```python
from build123d import *

# Parameters (mm, degrees)
SKETCH_1_W          = 70
SKETCH_1_H          = 50
SKETCH_1_R          = 1.6
EXTRUDE_1_DEPTH     = 3
SKETCH_2_W          = 30
SKETCH_2_H          = 30
CUT_EXTRUDE_1_DEPTH = 4
FILLET_1_R          = 5
SKETCH_3_W          = 30
SKETCH_3_H          = 6
EXTRUDE_2_DEPTH     = 3
FILLET_2_R          = 3


with BuildPart() as part:
    # 草图1 → 凸台-拉伸1 (new body)
    with BuildSketch(Plane.XY):
        Rectangle(SKETCH_1_W, SKETCH_1_H)
        with Locations((-25, -15)):
            Circle(SKETCH_1_R, mode=Mode.SUBTRACT)
        with Locations((-25, -5)):
            Circle(SKETCH_1_R, mode=Mode.SUBTRACT)
        with Locations((-25, 15)):
            Circle(SKETCH_1_R, mode=Mode.SUBTRACT)
        with Locations((-5, 15)):
            Circle(SKETCH_1_R, mode=Mode.SUBTRACT)
        with Locations((5, 15)):
            Circle(SKETCH_1_R, mode=Mode.SUBTRACT)
        with Locations((25, 15)):
            Circle(SKETCH_1_R, mode=Mode.SUBTRACT)
        with Locations((25, -5)):
            Circle(SKETCH_1_R, mode=Mode.SUBTRACT)
        with Locations((25, -15)):
            Circle(SKETCH_1_R, mode=Mode.SUBTRACT)
    extrude(amount=EXTRUDE_1_DEPTH)

    # 草图2 → 切除-拉伸1 (cut, through all)
    with BuildSketch(Plane.XY.offset(3)):
        with Locations((0, -10)):
            Rectangle(SKETCH_2_W, SKETCH_2_H)
    extrude(amount=-CUT_EXTRUDE_1_DEPTH, mode=Mode.SUBTRACT)

    # 圆角1
    fillet_1_edges = [part.edges().sort_by_distance(p)[0] for p in [
        (15, -25, 1.5),
        (-15, -25, 1.5),
        (-15, 5, 1.5),
        (15, 5, 1.5),
        (35, -25, 1.5),
        (-35, -25, 1.5),
        (-35, 25, 1.5),
        (35, 25, 1.5),
    ]]
    fillet(fillet_1_edges, radius=FILLET_1_R)

    # 草图3 → 凸台-拉伸2 (add)
    with BuildSketch(Plane.XY.offset(3)):
        with Locations((0, -13)):
            Rectangle(SKETCH_3_W, SKETCH_3_H)
    extrude(amount=-EXTRUDE_2_DEPTH)

    # 圆角2
    fillet_2_edges = [part.edges().sort_by_distance(p)[0] for p in [
        (-15, -16, 1.5),
        (-15, -10, 1.5),
        (15, -10, 1.5),
        (15, -16, 1.5),
    ]]
    fillet(fillet_2_edges, radius=FILLET_2_R)


solid = part.part
```
Read the model definition and answer for the solid it produces. Units are mm, in the model's axes. A direction names the side the tool comes from. Coordinates: 2 decimals unless noted, no trailing zeros. Write each loop counter-clockwise with the first axis right and the second up, starting at its lowest first coordinate (ties: lowest second). Pieces come first, ordered by that corner, then holes. Notation, with made-up numbers: (-21.75, 13) -> (20.25, 13) arc R35 cw to (20.25, 50) -> close; hole circle Ø11 at (-9, 24). An arc over 180 degrees is marked (long way). Return JSON: item names as keys, results as strings.
1. Determine the mould class of faces 1 (the face through (25, -25, 1)), 2 (the face through (23.82, 16.08, 1.48)), 3 (the face through (35, 0, 1)) for opening direction X: pulls with the +X half, pulls with the -X half, needs draft (parallel to the pull), parting line crosses it, or undercut.
Found:
{"face 1": "needs draft", "face 2": "undercut", "face 3": "pulls with the +X half"}
2. Each of these flat-tipped pins is pushed along its axis until it touches: P1, Ø5, axis at x = -5, y = 15, coming from the -Z side; P2, Ø1.5, axis at x = 1.5, z = 1, coming from the -Y side. Where does it stop, or does it pass through?
Found:
{"P1": "z = 0", "P2": "y = -16"}
3. A tool of negligible diameter and unlimited length cuts with its end or side. For faces 4 (the face through (14.14, -9.1, 1.48)), 5 (the face through (33, 24, 2)), 6 (the face through (0, -16, 2)), from which of +Z, -Z, +X, -X, +Y, -Y can it reach the whole face along a straight path? Write none if from no direction.
Found:
{"face 4": "+Z, -Z", "face 5": "+Z, -Z, +X, +Y", "face 6": "+Z, -Z, -Y"}
4. A cutting plane is placed at D-D (z = 2.2). Give the number of separate pieces and of enclosed holes in the cut face, and give its area (3 significant figures).
Found:
{"separate pieces": "1", "enclosed holes": "9", "area": "2,700 mm2"}
5. A cutting plane is placed at A-A (y = 15). Determine the outline of the cut face in (x, z), and give its area (3 significant figures).
Found:
{"outline": "(-35, 0) -> (-26.6, 0) -> (-26.6, 3) -> (-35, 3) -> close; (-23.4, 0) -> (-6.6, 0) -> (-6.6, 3) -> (-23.4, 3) -> close; (-3.4, 0) -> (3.4, 0) -> (3.4, 3) -> (-3.4, 3) -> close; (6.6, 0) -> (23.4, 0) -> (23.4, 3) -> (6.6, 3) -> close; (26.6, 0) -> (35, 0) -> (35, 3) -> (26.6, 3) -> close", "area": "172 mm2"}
6. Find the intervals of material crossed by line 1 along Y through (x, z) = (-25, 1.7); line 2 along Y through (x, z) = (5, 1.7); line 3 along Y through (x, z) = (-3, 2.8), in increasing order. Write a range as from..to.
Found:
{"line 1": "-25..-16.6, -13.4..-6.6, -3.4..13.4, 16.6..25", "line 2": "-16..-10, 5..13.4, 16.6..25", "line 3": "-16..-10, 5..25"}
7. A cutting plane is placed at B-B (x = -8.5). Determine the outline of the cut face in (y, z).
Found:
{"outline": "(-16, 0) -> (-10, 0) -> (-10, 3) -> (-16, 3) -> close; (5, 0) -> (25, 0) -> (25, 3) -> (5, 3) -> close"}
8. A cutting plane is placed at C-C (x = -25). Determine the outline of the cut face in (y, z).
Found:
{"outline": "(-25, 0) -> (-16.6, 0) -> (-16.6, 3) -> (-25, 3) -> close; (-13.4, 0) -> (-6.6, 0) -> (-6.6, 3) -> (-13.4, 3) -> close; (-3.4, 0) -> (13.4, 0) -> (13.4, 3) -> (-3.4, 3) -> close; (16.6, 0) -> (25, 0) -> (25, 3) -> (16.6, 3) -> close"}
